Answer from the drawing. Dimensions are ordinates in mm from the lowest x, y and z of the part. A direction names the side the tool comes from. Coordinates: 2 decimals unless noted, no trailing zeros. Order: outer loops, then holes, each group sorted by start corner. A loop starts at its lowest first (then second) coordinate and runs counter-clockwise, first axis right, second up. Notation, with made-up numbers: M 35,-15 L 66,-15 A31 ccw 66,16 Z; hole C 35,24.5 d4. An arc over 180 degrees is marked long. Write each question's results on one line, items separated by ' | '.
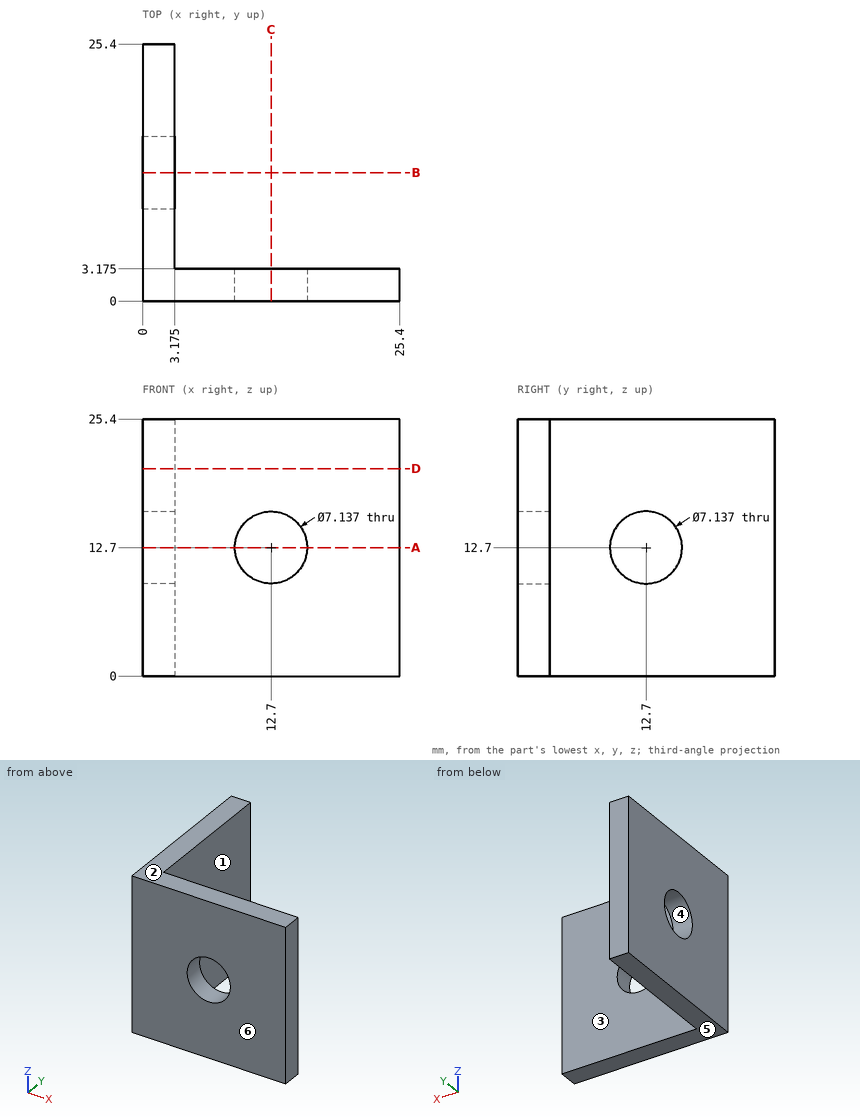
(1) Straight lines are drawn through the part: line 1 (Y direction, x = 1.4, z = 12.7); line 2 (Y direction, x = 6.75, z = 23.5) (1 decimal). For each, find the intervals that lie inside material, in ascending order.
Conclusion:
line 1: 0 to 9.13, 16.27 to 25.4 | line 2: 0 to 3.2
(2) The mould has two halves that part along Y. Classify the marked faces 3, 4, 5 and 6: pulls with the +Y half, pulls with the -Y half, needs draft (parallel to the pull), parting line crosses it, or undercut.
Conclusion:
face 3: pulls with the +Y half | face 4: undercut | face 5: needs draft | face 6: pulls with the -Y half
(3) For the marked faces 1 and 2, determine the directions among +Z, -Z, +X, -X, +Y, -Y from which every point of the face is accessible in a straight line to the end or side of a thin tool.
Conclusion:
face 1: +Z, -Z, +X, +Y | face 2: +Z, +X, -X, +Y, -Y
(4) Given pin 1 (6 mm diameter, centred on y = 19.5, z = 15.5, fed in from +X) (3 decimals); pin 2 (11 mm diameter, centred on x = 19.5, z = 8.5, fed in from +Y) (3 decimals), each flat-ended and moving along its own axis, determine where each tip first touches the part or whether it passes through.
Conclusion:
pin 1: x = 3.175 | pin 2: y = 3.175
(5) The part is cut by section B-B, the plane y = 12.7. Write down the section's boundary in (x, z) (1 decimal).
Conclusion:
outline: M 0,0 L 3.2,0 L 3.2,9.1 L 0,9.1 Z; M 0,16.3 L 3.2,16.3 L 3.2,25.4 L 0,25.4 Z
(6) The part is cut by section A-A, the plane z = 12.7. Write down the section's boundary in (x, y) (1 decimal).
Conclusion:
outline: M 0,0 L 9.1,0 L 9.1,3.2 L 3.2,3.2 L 3.2,9.1 L 0,9.1 Z; M 0,16.3 L 3.2,16.3 L 3.2,25.4 L 0,25.4 Z; M 16.3,0 L 25.4,0 L 25.4,3.2 L 16.3,3.2 Z
(7) The part is cut by section D-D, the plane z = 20.5. Write down the section's boundary in (x, y) (1 decimal).
Conclusion:
outline: M 0,0 L 25.4,0 L 25.4,3.2 L 3.2,3.2 L 3.2,25.4 L 0,25.4 Z
